Drawing for the job (mm, zero at the part's lowest x, y, z). Give positions to 0.01 mm unless a question says otherwise; leave off trailing zeros. Order: outer loops, then holes, each group sorted by start corner. A loop starts at its lowest first (then second) coordinate and runs counter-clockwise, first axis right, second up. Notation, with made-up numbers: M 26.5,65.5 L 54.5,65.5 A6 cw 54.5,75.5 Z; hole C 87.25,-21 d2. An arc over 180 degrees is marked long. Answer as a JSON object with one key per item and string values.
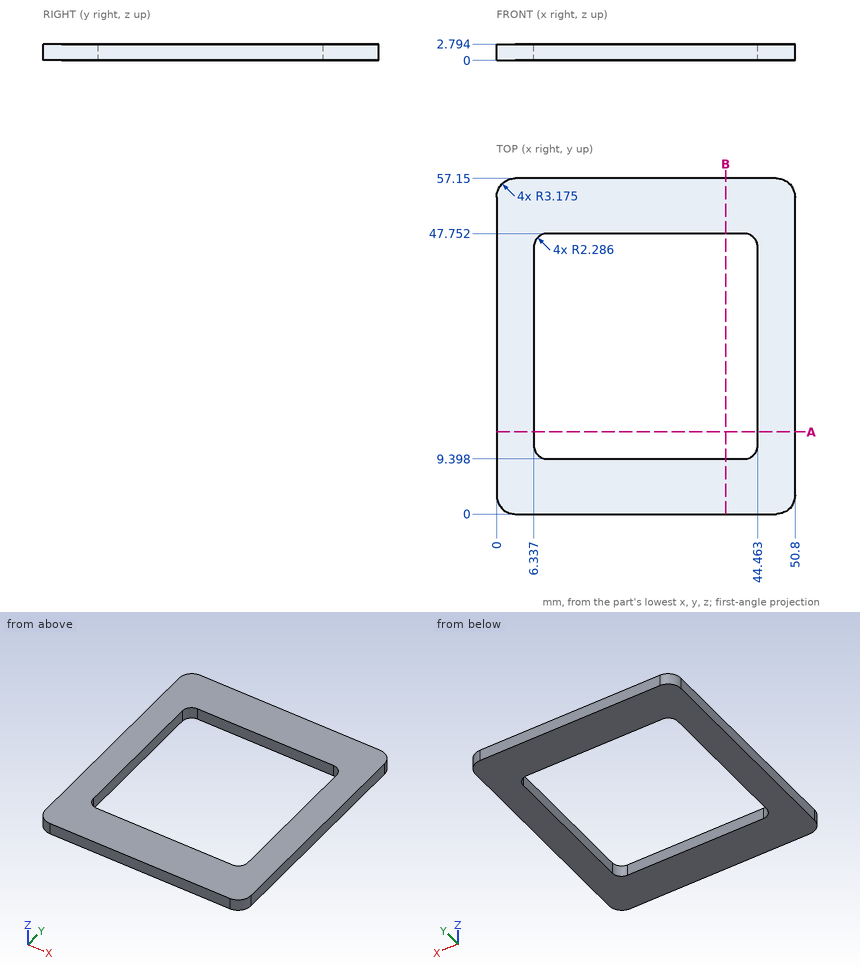
1. Cut at A-A on y = 14. Give the cut face in (x, z).
Worked answers:
{"outline": "M 0,0 L 6.34,0 L 6.34,2.79 L 0,2.79 Z; M 44.46,0 L 50.8,0 L 50.8,2.79 L 44.46,2.79 Z"}
2. Cut at B-B on x = 39. Give the cut face in (y, z), plus the area to 3 significant figures.
Worked answers:
{"outline": "M 0,0 L 9.4,0 L 9.4,2.79 L 0,2.79 Z; M 47.75,0 L 57.15,0 L 57.15,2.79 L 47.75,2.79 Z", "area": "52.5 mm^2"}
3. Probe line 1 along Y through (x, z) = (27, 2.4); line 2 along X through (y, z) = (34, 1.95); line 3 along Y through (x, z) = (42.5, 0.9). List the from-to ranges inside material, lowest first.
Worked answers:
{"line 1": "y = 0 to 9.4, 47.75 to 57.15", "line 2": "x = 0 to 6.34, 44.46 to 50.8", "line 3": "y = 0 to 9.42, 47.73 to 57.15"}
